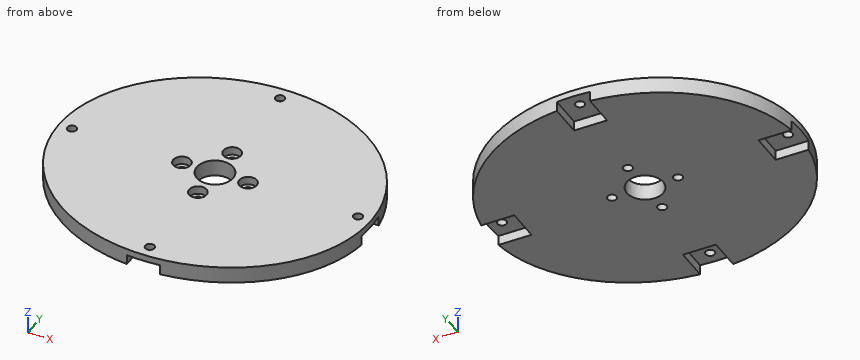
from build123d import *

# Parameters (mm, degrees)
SKETCH1_RX          = 47.3
SKETCH1_RY          = 42
SKETCH1_R           = 5.5
SKETCH1_R_2         = 1.4
BOSS_EXTRUDE1_DEPTH = 5
CUT_EXTRUDE3_START  = -2.5
SKETCH5_R           = 2.65
SKETCH5_R_2         = 1.4
CUT_EXTRUDE3_DEPTH  = 2.5
CUT_EXTRUDE4_DEPTH  = 3


with BuildPart() as part:
    # Sketch1 → Boss-Extrude1 (new body)
    with BuildSketch(Plane.XY):
        with Locations(Location((0, 0), (0, 0, 180))):
            Ellipse(SKETCH1_RX, SKETCH1_RY)
        Circle(SKETCH1_R, mode=Mode.SUBTRACT)
        with Locations((-10, 0)):
            Circle(SKETCH1_R_2, mode=Mode.SUBTRACT)
        with Locations((0, 10)):
            Circle(SKETCH1_R_2, mode=Mode.SUBTRACT)
        with Locations((10, 0)):
            Circle(SKETCH1_R_2, mode=Mode.SUBTRACT)
        with Locations((0, -10)):
            Circle(SKETCH1_R_2, mode=Mode.SUBTRACT)
        with Locations((0, 38)):
            Circle(SKETCH1_R_2, mode=Mode.SUBTRACT)
        with Locations((-43.3, 0)):
            Circle(SKETCH1_R_2, mode=Mode.SUBTRACT)
        with Locations(Location((43.3, 0, 0), (0, 0, 180))):
            Circle(SKETCH1_R_2, mode=Mode.SUBTRACT)
        with Locations(Location((0, -38, 0), (0, 0, 180))):
            Circle(SKETCH1_R_2, mode=Mode.SUBTRACT)
    extrude(amount=BOSS_EXTRUDE1_DEPTH)

    # Sketch5 → Cut-Extrude3 (cut)
    # profile 1 of 4: a face of its own
    with BuildSketch(Plane.XY.offset(5).offset(CUT_EXTRUDE3_START)):
        with Locations((0, 10)):
            Circle(SKETCH5_R)
        with Locations((0, 10)):
            Circle(SKETCH5_R_2, mode=Mode.SUBTRACT)
    # profile 2 of 4: a face of its own
    with BuildSketch(Plane.XY.offset(5).offset(CUT_EXTRUDE3_START)):
        with Locations((10, 0)):
            Circle(SKETCH5_R)
        with Locations((10, 0)):
            Circle(SKETCH5_R_2, mode=Mode.SUBTRACT)
    # profile 3 of 4: a face of its own
    with BuildSketch(Plane.XY.offset(5).offset(CUT_EXTRUDE3_START)):
        with Locations((0, -10)):
            Circle(SKETCH5_R)
        with Locations((0, -10)):
            Circle(SKETCH5_R_2, mode=Mode.SUBTRACT)
    # profile 4 of 4: a face of its own
    with BuildSketch(Plane.XY.offset(5).offset(CUT_EXTRUDE3_START)):
        with Locations((-10, 0)):
            Circle(SKETCH5_R)
        with Locations((-10, 0)):
            Circle(SKETCH5_R_2, mode=Mode.SUBTRACT)
    extrude(amount=CUT_EXTRUDE3_DEPTH, mode=Mode.SUBTRACT)

    # Sketch6 → Cut-Extrude4 (cut)
    with BuildSketch(Plane(origin=(0, 0, 0), x_dir=(-1, 0, 0), z_dir=(0, 0, -1))):
        with BuildLine():
            Line((-5, 41.764681883), (-5, 31.764681883))
            Line((-5, 31.764681883), (5, 31.764681883))
            Line((5, 31.764681883), (5, 41.764681883))
            add(Edge.make_bspline(
                [(5, 41.764681883), (0, 42.236643989), (-5, 41.764681883)],
                knots=[1.464890217, 1.464890217, 1.464890217, 1.676702437, 1.676702437, 1.676702437], degree=2, weights=[1, 0.994397188, 1]))
        make_face()
        with BuildLine():
            Line((-46.963628217, 5), (-36.963628217, 5))
            Line((-36.963628217, 5), (-36.963628217, -5))
            Line((-36.963628217, -5), (-46.963628217, -5))
            add(Edge.make_bspline(
                [(-46.963628217, 5), (-47.638781009, 0), (-46.963628217, -5)],
                knots=[3.022262029, 3.022262029, 3.022262029, 3.260923278, 3.260923278, 3.260923278], degree=2, weights=[1, 0.992888546, 1]))
        make_face()
        with BuildLine():
            Line((46.963628217, 5), (36.963628217, 5))
            Line((36.963628217, 5), (36.963628217, -5))
            Line((36.963628217, -5), (46.963628217, -5))
            add(Edge.make_bspline(
                [(46.963628217, -5), (47.638781009, 0), (46.963628217, 5)],
                knots=[3.022262029, 3.022262029, 3.022262029, 3.260923278, 3.260923278, 3.260923278], degree=2, weights=[1, 0.992888546, 1]))
        make_face()
        with BuildLine():
            Line((5, -31.764681883), (5, -41.764681883))
            add(Edge.make_bspline(
                [(-5, -41.764681883), (0, -42.236643989), (5, -41.764681883)],
                knots=[4.60648287, 4.60648287, 4.60648287, 4.81829509, 4.81829509, 4.81829509], degree=2, weights=[1, 0.994397188, 1]))
            Line((-5, -41.764681883), (-5, -31.764681883))
            Line((-5, -31.764681883), (5, -31.764681883))
        make_face()
    extrude(amount=-CUT_EXTRUDE4_DEPTH, mode=Mode.SUBTRACT)


solid = part.part
Geometry: final body of the model. Coordinates: model frame, mm. Round coordinates to 2 decimals unless told otherwise and drop trailing zeros. Put each result on its own line as item: value. Start each with the question number.
Q1. Section A-A on y = 0. Give the number of separate pieces and of enclosed holes in the cut face, and give its area (3 significant figures).
Q2. First-contact query: pin 1 (1 mm diameter, centred on x = -11, z = 4, fed in from -Y); pin 2 (2.5 mm diameter, centred on y = -38, z = 1.5, fed in from +X); pin 3 (3 mm diameter, centred on x = -10, y = 0, fed in from +Z). Flat tips, straight axial feed; report the tip coordinate or a pass-through.
Q3. Line query: probe 1 along Y at (x, z) = (0, 3.85); probe 2 along Z at (x, y) = (42.5, 4.5); probe 3 along Y at (x, z) = (38, 2.3). Output: solid intervals per line, ascending.
Ans:
1. separate pieces: 6
1. enclosed holes: 0
1. area: 304 mm2
2. pin 1: stops at y = -40.95
2. pin 2: stops at x = 22.9
2. pin 3: stops at z = 2.5
3. probe 1: y = -42 to -39.4, -36.6 to -12.65, -7.35 to -5.5, 5.5 to 7.35, 12.65 to 36.6, 39.4 to 42
3. probe 2: z = 3 to 5
3. probe 3: y = -25.01 to -5, 5 to 25.01
